Verification items for the finished model (mm, model axes). Face numbers are marked on the shaded views. A direction names the side the tool comes from. Round coordinates to 2 decimals unless told otherwise and drop trailing zeros. Write each loop counter-clockwise with the first axis right and the second up, starting at its lowest first coordinate (ties: lowest second). Pieces come first, ordered by that corner, then holes. Notation, with made-up numbers: (-31.75, -11) - (-21.75, -11) arc R33 ccw to (-21.75, 18) - close; hole circle Ø6 at (50, 53). An arc over 180 degrees is marked (long way). Answer as a JSON object with one key per item and string values.
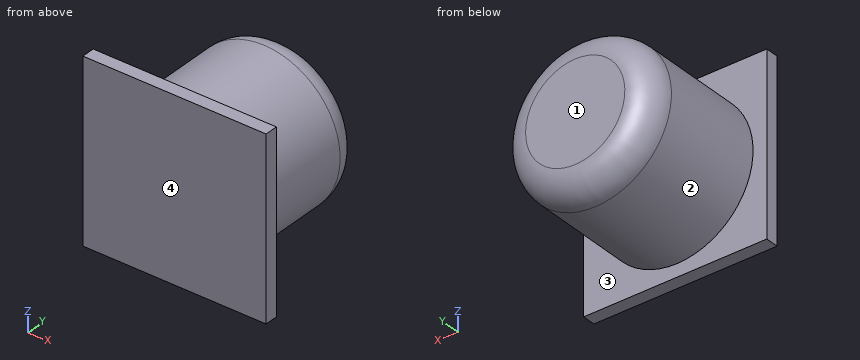
```python
from build123d import *

# Parameters (mm, degrees)
SKETCH2_R           = 2.9
BOSS_EXTRUDE1_DEPTH = 0.5
BOSS_EXTRUDE2_START = 5
SKETCH3_R           = 2.9
BOSS_EXTRUDE2_DEPTH = 5
SKETCH4_W           = 7.010834482
SKETCH4_H           = 6.831005896
BOSS_EXTRUDE3_DEPTH = 0.5
FILLET1_R           = 1


with BuildPart() as part:
    # Sketch2 → Boss-Extrude1 (new body)
    with BuildSketch(Plane(origin=(0, 0, 0), x_dir=(1, 0, 0), z_dir=(0, 1, 0))):
        with Locations(Location((0, 0, 0), (0, 0, 270))):
            Circle(SKETCH2_R)
    extrude(amount=-BOSS_EXTRUDE1_DEPTH)

    # Sketch3 → Boss-Extrude2 (add)
    with BuildSketch(Plane(origin=(0, 0, 0), x_dir=(1, 0, 0), z_dir=(0, 1, 0)).offset(BOSS_EXTRUDE2_START)):
        with Locations(Location((0, 0, 0), (0, 0, 270))):
            Circle(SKETCH3_R)
    extrude(amount=-BOSS_EXTRUDE2_DEPTH)

    # Sketch4 → Boss-Extrude3 (add)
    with BuildSketch(Plane(origin=(0, 0, 0), x_dir=(1, 0, 0), z_dir=(0, 1, 0))):
        with Locations((0.077133625, -0.02775209)):
            Rectangle(SKETCH4_W, SKETCH4_H)
    extrude(amount=-BOSS_EXTRUDE3_DEPTH)

    # Fillet1
    fillet1_edges = [part.edges().sort_by_distance(p)[0] for p in [
        (0, 5, -2.9),
    ]]
    fillet(fillet1_edges, radius=FILLET1_R)


solid = part.part
```
1. Go/stop test with a flat-tipped pin: pin 1 (2 mm diameter, centred on x = 0, y = 4, fed in from +Z). Record where the tip stops, or that it passes through.
Completed:
{"pin 1": "stops at z = 2.9"}
2. Cross-section at D-D (y = 4.7). Record the boundary of the cut face in (x, z).
Completed:
{"outline": "circle Ø5.23 at (0, 0)"}
3. Access from +Z, -Z, +X, -X, +Y, -Y to the whole of each face (thin tool, end or side, straight path). Record for the marked faces 3 and 4.
Completed:
{"face 3": "+Y", "face 4": "+Z, -Z, +X, -X, -Y"}
4. Mould release check, pull along Z, two halves, no side actions. Record for the marked faces 1 and 2: released by +Z, released by -Z, zero draft, split by the parting line, or undercut.
Completed:
{"face 1": "zero draft", "face 2": "split by the parting line"}
5. Cross-section at A-A (z = 0). Record the boundary of the cut face in (x, y).
Completed:
{"outline": "(-3.43, -0.5) - (3.58, -0.5) - (3.58, 0) - (2.9, 0) - (2.9, 4) arc R1 ccw to (1.9, 5) - (-1.9, 5) arc R1 ccw to (-2.9, 4) - (-2.9, 0) - (-3.43, 0) - close"}
6. Material ranges on probe 1 along Y at (x, z) = (-2, 2.75); probe 2 along X at (y, z) = (2, 0); probe 3 along X at (y, z) = (0.95, 1), recorded low to high. Write a range as from..to.
Completed:
{"probe 1": "y = -0.5..0", "probe 2": "x = -2.9..2.9", "probe 3": "x = -2.72..2.72"}
7. Cross-section at C-C (y = 2.7). Record the boundary of the cut face in (x, z).
Completed:
{"outline": "circle Ø5.8 at (0, 0)"}
8. Cross-section at B-B (x = 0). Record the boundary of the cut face in (y, z).
Completed:
{"outline": "(-0.5, -3.39) - (0, -3.39) - (0, -2.9) - (4, -2.9) arc R1 ccw to (5, -1.9) - (5, 1.9) arc R1 ccw to (4, 2.9) - (0, 2.9) - (0, 3.44) - (-0.5, 3.44) - close"}
